Model file for the job. Use its own axes, mm. Give positions to 0.01 mm unless a question says otherwise; leave off trailing zeros. Loops run counter-clockwise (first coordinate to the right, second up) from the corner with the lowest first, then second, coordinate; pieces in that order, holes last. Notation, with made-up numbers: M 17,88.25 L 40,88.25 A30 cw 40,123.25 Z; hole C 22.25,36.5 d1. An arc over 180 degrees is marked long. Answer in a Markdown table with one row per item.
```python
from build123d import *

# Parameters (mm, degrees)
SKETCH1_R           = 1.6999966
SKETCH1_R_2         = 4
BOSS_EXTRUDE1_DEPTH = 1.5875


with BuildPart() as part:
    # Sketch1 → Boss-Extrude1 (new body)
    with BuildSketch(Plane(origin=(0, 0, 0), x_dir=(1, 0, 0), z_dir=(0, 1, 0))):
        with BuildLine():
            Line((-9.525, 15.875), (9.525, 15.875))
            ThreePointArc((9.525, 15.875), (14.015128061, 14.015128061), (15.875, 9.525))
            Line((15.875, 9.525), (15.875, -9.525))
            ThreePointArc((15.875, -9.525), (14.015128061, -14.015128061), (9.525, -15.875))
            Line((9.525, -15.875), (-9.525, -15.875))
            ThreePointArc((-9.525, -15.875), (-14.015128061, -14.015128061), (-15.875, -9.525))
            Line((-15.875, -9.525), (-15.875, 9.525))
            ThreePointArc((-15.875, 9.525), (-14.015128061, 14.015128061), (-9.525, 15.875))
        make_face()
        with Locations((-6.735192091, -6.735192091)):
            Circle(SKETCH1_R, mode=Mode.SUBTRACT)
        with Locations((6.735192091, -6.735192091)):
            Circle(SKETCH1_R, mode=Mode.SUBTRACT)
        Circle(SKETCH1_R_2, mode=Mode.SUBTRACT)
        with Locations((6.735192091, 6.735192091)):
            Circle(SKETCH1_R, mode=Mode.SUBTRACT)
        with Locations((-6.735192091, 6.735192091)):
            Circle(SKETCH1_R, mode=Mode.SUBTRACT)
    extrude(amount=BOSS_EXTRUDE1_DEPTH)


solid = part.part
```
(1) Mould opens along X. For faces 1 (the flat face through (-3, 0, 3)), 2 (the cylindrical face through (-5.1, 0.8, -7.2)), 3 (the flat face through (-15.875, 1, 0)) say: pulls with the +X half, pulls with the -X half, needs draft (parallel to the pull), parting line crosses it, or undercut.
Established:
| item | result |
|---|---|
| face 1 | needs draft |
| face 2 | undercut |
| face 3 | pulls with the -X half |
(2) Saw through at A-A, the plane z = 0. Give the cut face in (x, y) (1 decimal), and give its area (3 significant figures).
Established:
| item | result |
|---|---|
| outline | M -15.9,0 L -4,0 L -4,1.6 L -15.9,1.6 Z; M 4,0 L 15.9,0 L 15.9,1.6 L 4,1.6 Z |
| area | 37.7 mm2 |
(3) Saw through at C-C, the plane x = -8. Give the cut face in (y, z) (1 decimal), and give its area (3 significant figures).
Established:
| item | result |
|---|---|
| outline | M 0,-15.9 L 1.6,-15.9 L 1.6,-7.9 L 0,-7.9 Z; M 0,-5.6 L 1.6,-5.6 L 1.6,5.6 L 0,5.6 Z; M 0,7.9 L 1.6,7.9 L 1.6,15.9 L 0,15.9 Z |
| area | 43.2 mm2 |
(4) Wall check: L1, parallel to Z at x = -8, y = 0.3 (3 decimals); L2, parallel to Z at x = 7.5, y = 1.4 (3 decimals); L3, parallel to Z at x = 0, y = 0.5 (3 decimals). Give the ranges that are in metal, low to high.
Established:
| item | result |
|---|---|
| L1 | z = -15.875 to -7.871, -5.599 to 5.599, 7.871 to 15.875 |
| L2 | z = -15.875 to -8.253, -5.217 to 5.217, 8.253 to 15.875 |
| L3 | z = -15.875 to -4, 4 to 15.875 |
(5) Flat gauge pins, fed straight in: P1, Ø2, axis at x = 6.74, z = 6.74, coming from the -Y side; P2, Ø4, axis at x = -6.74, z = 6.74, coming from the -Y side. Where does each tip first touch, or does it go through?
Established:
| item | result |
|---|---|
| P1 | passes through |
| P2 | stops at y = 0 |
(6) Saw through at B-B, the plane x = 0. Give the cut face in (y, z) (1 decimal), and give its area (3 significant figures).
Established:
| item | result |
|---|---|
| outline | M 0,-15.9 L 1.6,-15.9 L 1.6,-4 L 0,-4 Z; M 0,4 L 1.6,4 L 1.6,15.9 L 0,15.9 Z |
| area | 37.7 mm2 |
(7) Saw through at D-D, the plane y = 1. Give the cut face in (x, z) (3 decimals).
Established:
| item | result |
|---|---|
| outline | M -15.875,-9.525 A6.35 ccw -9.525,-15.875 L 9.525,-15.875 A6.35 ccw 15.875,-9.525 L 15.875,9.525 A6.35 ccw 9.525,15.875 L -9.525,15.875 A6.35 ccw -15.875,9.525 Z; hole C -6.735,-6.735 d3.4; hole C -6.735,6.735 d3.4; hole C 0,0 d8; hole C 6.735,-6.735 d3.4; hole C 6.735,6.735 d3.4 |
